Geometry: final body of the model. Coordinates: model frame, mm. A direction names the side the tool comes from. Give positions to 0.01 mm unless a question says otherwise; leave off trailing zeros. Write each loop counter-clockwise with the first axis right and the second up, starting at its lowest first coordinate (ties: lowest second). Pieces come first, ordered by that corner, then holes. Notation, with made-up numbers: (43, 83.5) - (84, 83.5) arc R23 cw to (84, 122.5) - close; hole circle Ø1 at (2, 72.25). An arc over 180 degrees is marked (long way). Return JSON: item names as keys, results as strings.
from build123d import *

# Parameters (mm, degrees)
ESQUISSE1_R             = 1.7
ESQUISSE1_R_2           = 1.8
ESQUISSE1_R_3           = 4.2
BOSS_EXTRU_1_DEPTH      = 2
ESQUISSE2_R             = 1.9
ENL_V_MAT_EXTRU_1_DEPTH = 1.2
ESQUISSE4_W             = 2.8
ESQUISSE4_H             = 11
BOSS_EXTRU_3_DEPTH      = 1
CONG_1_R                = 0.5


with BuildPart() as part:
    # Esquisse1 → Boss.-Extru.1 (new body)
    with BuildSketch(Plane(origin=(0, 0, 0), x_dir=(1, 0, 0), z_dir=(0, 1, 0))):
        Polygon((10, 16.4), (-10, 16.4), (-10, -6), (6, -6), (6, 5), (10, 5), align=None)
        with Locations((-7, -3.5)):
            Circle(ESQUISSE1_R, mode=Mode.SUBTRACT)
        with Locations((-7, 1)):
            Circle(ESQUISSE1_R_2, mode=Mode.SUBTRACT)
        Circle(ESQUISSE1_R_3, mode=Mode.SUBTRACT)
        Polygon((-6.4, 12.9), (-6.4, 14.4), (6.4, 14.4), (6.4, 12.9), (8, 12.9), (8, 9.5), (6.4, 9.5), (6.4, 8), (-6.4, 8), (-6.4, 9.5), (-8, 9.5), (-8, 12.9), align=None, mode=Mode.SUBTRACT)
    extrude(amount=BOSS_EXTRU_1_DEPTH)

    # Esquisse2 → Enlèv. mat.-Extru.1 (cut)
    with BuildSketch(Plane(origin=(0, 2, 0), x_dir=(1, 0, 0), z_dir=(0, 1, 0))):
        with Locations((-7, 5.5)):
            Circle(ESQUISSE2_R)
    extrude(amount=-ENL_V_MAT_EXTRU_1_DEPTH, mode=Mode.SUBTRACT)

    # Esquisse4 → Boss.-Extru.3 (add)
    with BuildSketch(Plane.XZ):
        with Locations((7.4, 0.5)):
            Rectangle(ESQUISSE4_W, ESQUISSE4_H)
    extrude(amount=-BOSS_EXTRU_3_DEPTH)

    # Congé1
    cong_1_edges = [part.edges().sort_by_distance(p)[0] for p in [
        (-10, 1, 6),
        (-10, 1, -16.4),
        (10, 1, -16.4),
    ]]
    fillet(cong_1_edges, radius=CONG_1_R)


solid = part.part
Q1. Section query C-C, the plane x = 0. Return the cut outline in (y, z).
Answer key:
{"outline": "(0, -16.4) - (2, -16.4) - (2, -14.4) - (0, -14.4) - close; (0, -8) - (2, -8) - (2, -4.2) - (0, -4.2) - close; (0, 4.2) - (2, 4.2) - (2, 6) - (0, 6) - close"}
Q2. Section query B-B, the plane y = 0.4. Return the cut outline in (x, z).
Answer key:
{"outline": "(-10, -15.9) arc R0.5 ccw to (-9.5, -16.4) - (9.5, -16.4) arc R0.5 ccw to (10, -15.9) - (10, -5) - (8.8, -5) - (8.8, 6) - (-9.5, 6) arc R0.5 ccw to (-10, 5.5) - close; hole circle Ø3.6 at (-7, -1); hole circle Ø3.4 at (-7, 3.5); hole (-8, -12.9) - (-6.4, -12.9) - (-6.4, -14.4) - (6.4, -14.4) - (6.4, -12.9) - (8, -12.9) - (8, -9.5) - (6.4, -9.5) - (6.4, -8) - (-6.4, -8) - (-6.4, -9.5) - (-8, -9.5) - close; hole circle Ø8.4 at (0, 0)"}
Q3. Set-up query: faces 1 (the flat face through (8.8, 0.5, 0.4)), 2 (the flat face through (8, 1, -11)), 3 (the flat face through (7, 1, 1)). Return all of +Z, -Z, +X, -X, +Y, -Y with unobstructed straight access to the full face (end or side cutting, diameter ignored); none if empty.
Answer key:
{"face 1": "+Z, +X, +Y, -Y", "face 2": "+Y, -Y", "face 3": "+Z, +X, +Y"}
Q4. Mould query, pull axis X, two halves, no side actions, for faces 4 (the cylindrical face through (-8.4, 1.408, -6.784)), 5 (the flat face through (0, 0, -5)), 6 (the flat face through (10, 1, -10)). Classes: pulls with the +X half, pulls with the -X half, needs draft (parallel to the pull), parting line crosses it, or undercut.
Answer key:
{"face 4": "undercut", "face 5": "needs draft", "face 6": "pulls with the +X half"}
Q5. Section query D-D, the plane z = 3.5. Return the cut outline in (x, y), plus the area to 3 significant figures.
Answer key:
{"outline": "(-10, 0) - (-8.7, 0) - (-8.7, 2) - (-10, 2) - close; (-5.3, 0) - (-2.32, 0) - (-2.32, 2) - (-5.3, 2) - close; (2.32, 0) - (8.8, 0) - (8.8, 1) - (6, 1) - (6, 2) - (2.32, 2) - close", "area": "18.7 mm^2"}
Q6. Material intervals for probe 1 along Z at (x, y) = (0, 0.45); probe 2 along Z at (x, y) = (-7, 1.5); probe 3 along X at (y, z) = (1.7, -5.5), sorted ascending. Write a range as [from, to].
Answer key:
{"probe 1": "z = [-16.4, -14.4], [-8, -4.2], [4.2, 6]", "probe 2": "z = [-16.4, -12.9], [-9.5, -7.4], [-3.6, -2.8], [0.8, 1.8], [5.2, 6]", "probe 3": "x = [-10, -8.9], [-5.1, 10]"}
Q7. Pin query (flat end, axial travel): P1, Ø0.8, axis at x = 7, z = -0.5, coming from the +Y side. Return the tip coordinate at first contact, or that it passes through.
Answer key:
{"P1": "stops at y = 1"}
Q8. Section query A-A, the plane x = -7. Return the cut outline in (y, z).
Answer key:
{"outline": "(0, -16.4) - (2, -16.4) - (2, -12.9) - (0, -12.9) - close; (0, -9.5) - (2, -9.5) - (2, -7.4) - (0.8, -7.4) - (0.8, -3.6) - (2, -3.6) - (2, -2.8) - (0, -2.8) - close; (0, 0.8) - (2, 0.8) - (2, 1.8) - (0, 1.8) - close; (0, 5.2) - (2, 5.2) - (2, 6) - (0, 6) - close"}
